Could you check a few things on this model? Use its own coordinates, in mm. Face numbers are marked on the shaded views. A direction names the side the tool comes from. Give positions to 0.01 mm unless a question says otherwise; leave off trailing zeros. Use a Markdown table: item, result. Add a question column.
1) If I drill on line 1 along X through (y, z) = (0, -11.25); line 2 along X through (y, z) = (-11.5, -2.25); line 3 along Y through (x, z) = (-4, -1.5), over which ranges is the centre line in solid material (lowest first)? Write a range as [from, to].
2) Will these pins go through, and if not, where does the flat tip stop? pin 1 Ø2 at (x, z) = (-6, -16) entering from +Y; pin 2 Ø3 at (x, z) = (16.5, -2.5) entering from +Y; pin 3 Ø1.1 at (x, z) = (-15, -2) entering from +Y; pin 4 Ø15 at (x, y) = (0, 0) entering from +Z.
3) We'd pull the mould along Y, two halves only. Please class the marked faces 5, 6, 7 and 8: +Y half, -Y half, draft (parallel to the pull), parting line (faces both ways), or undercut.
4) Suppose I cut it at A-A on z = -4.25. Count the separate pieces of the cut face and the enclosed holes in it, and give its area (3 significant figures).
5) Which directions (+Z, -Z, +X, -X, +Y, -Y) give clear straight access to the entire face, cutting with the end or side of a thin tool? Please do the marked faces 1, 2, 3 and 4.
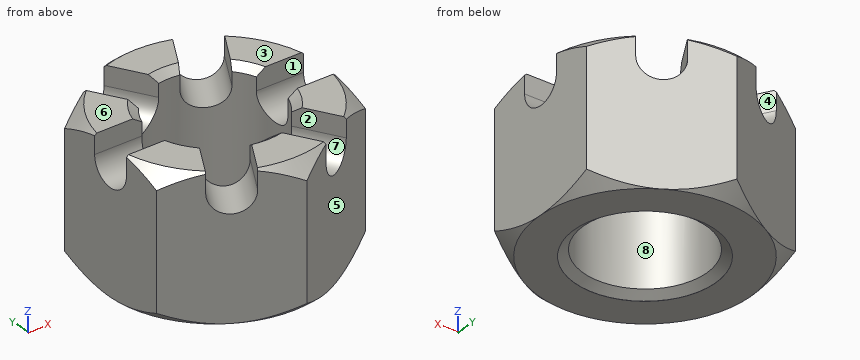
```python
from build123d import *

# Parameters (mm, degrees)
BASENUT_START     = -25.8572
BASENUTSKE_R      = 11.1125
BASENUT_DEPTH     = 25.8572
SLOT_DEPTH        = 52.030136114
SLOTPATTERN_COUNT = 3
SLOTPATTERN_ANGLE = 120


with BuildPart() as part:
    # BaseNutSke → BaseNut (new body)
    with BuildSketch(Plane.XY.offset(BASENUT_START)):
        Polygon((19.05, 10.998522628), (19.05, -10.998522628), (0, -21.997045256), (-19.05, -10.998522628), (-19.05, 10.998522628), (0, 21.997045256), align=None)
        Circle(BASENUTSKE_R, mode=Mode.SUBTRACT)
    extrude(amount=BASENUT_DEPTH)

    # Sketch4 → Slot (cut, through all)
    with BuildSketch(Plane(origin=(19.05, 0, 0), x_dir=(0, 0, -1), z_dir=(1, 0, 0))):
        with BuildLine():
            Line((3.5052, 3.81), (0, 3.81))
            Line((0, 3.81), (0, -3.81))
            Line((0, -3.81), (3.5052, -3.81))
            ThreePointArc((3.5052, -3.81), (7.3152, 0), (3.5052, 3.81))
        make_face()
    slot = extrude(amount=-SLOT_DEPTH, mode=Mode.SUBTRACT)

    # SlotPattern: Slot ×3 about axis
    slotpattern_axis = Axis((0, 0, 0), (0, 0, 1))
    for i in range(1, SLOTPATTERN_COUNT):
        add(slot.rotate(slotpattern_axis, i * SLOTPATTERN_ANGLE / (SLOTPATTERN_COUNT - 1)), mode=Mode.SUBTRACT)

    # Sketch3 → Double-Chamfer (revolve, cut)
    with BuildSketch(Plane(origin=(0, 0, 0), x_dir=(0, 0, -1), z_dir=(1, 0, 0)), mode=Mode.PRIVATE) as double_chamfer_sk:
        Polygon((25.8572, 19.05), (23.3172, 21.997045256), (23.3172, 34.697045256), (38.5572, 34.697045256), (38.5572, 19.05), align=None)
        Polygon((2.54, 21.997045256), (2.54, 34.697045256), (-12.7, 34.697045256), (-12.7, 19.05), (0, 19.05), align=None)
    revolve(double_chamfer_sk.sketch.rotate(Axis((0, 0, 0), (0, 0, -1)), 90), axis=Axis((0, 0, 0), (0, 0, -1)), mode=Mode.SUBTRACT)

    # EndChamferSketch → EndChamfer (revolve, cut)
    with BuildSketch(Plane(origin=(0, 0, 0), x_dir=(0, 0, -1), z_dir=(1, 0, 0)), mode=Mode.PRIVATE) as endchamfer_sk:
        Polygon((25.8318, 12.7), (24.609062586, 10.95375), (25.8826, 10.95375), (25.8826, 12.7), align=None)
        Polygon((-0.0508, 12.7), (0, 12.7), (1.222737414, 10.95375), (-0.0508, 10.95375), align=None)
    revolve(endchamfer_sk.sketch.rotate(Axis((0, 0, -25.037505729), (0, 0, -1)), 270), axis=Axis((0, 0, -25.037505729), (0, 0, -1)), mode=Mode.SUBTRACT)


solid = part.part
```
Answer block:
| question | item | result |
|---|---|---|
| 1 | line 1 | x = [-19.05, -11.11], [11.11, 19.05] |
| 1 | line 2 | x = [-18.18, -11.04], [-2.24, 2.24], [11.04, 18.18] |
| 1 | line 3 | y = [-19.69, -14.55], [14.55, 19.69] |
| 2 | pin 1 | stops at y = 19.11 |
| 2 | pin 2 | stops at y = 13.34 |
| 2 | pin 3 | stops at y = 13.65 |
| 2 | pin 4 | passes through |
| 3 | face 5 | -Y half |
| 3 | face 6 | draft |
| 3 | face 7 | undercut |
| 3 | face 8 | undercut |
| 4 | separate pieces | 6 |
| 4 | enclosed holes | 0 |
| 4 | area | 504 mm^2 |
| 5 | face 1 | +Z, +X, -X |
| 5 | face 2 | +Z, -Y |
| 5 | face 3 | +Z, +X, -X, +Y, -Y |
| 5 | face 4 | +Z, +Y |
